Design review of the part built by this model. Coordinates are the model's own, in mm. Face numbers are marked on the shaded views. A direction names the side the tool comes from. Give positions to 0.01 mm unless a question says otherwise; leave off trailing zeros. Write each loop counter-clockwise with the first axis right and the second up, starting at its lowest first coordinate (ties: lowest second). Pieces come first, ordered by that corner, then holes. Notation, with made-up numbers: (89.25, 63.25) -> (99.25, 63.25) arc R22 ccw to (99.25, 97.25) -> close; hole circle Ø5 at (-33.5, 33.25). An arc over 180 degrees is marked (long way). Use CSV: the item, a comma, the result in double quotes.
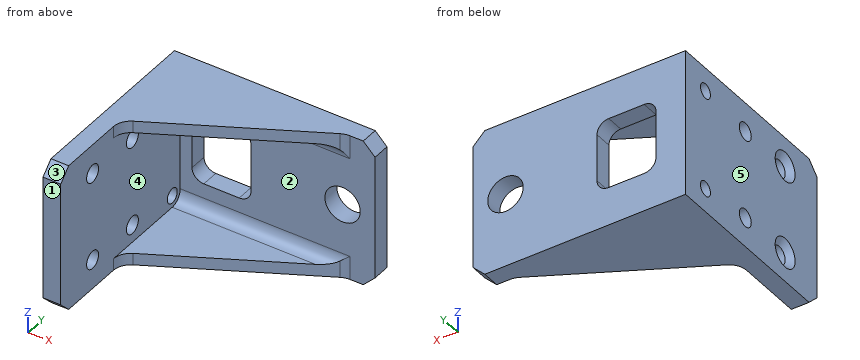
```python
from build123d import *

# Parameters (mm, degrees)
EXTRUDE_1_DEPTH     = 25
SKETCH_2_R          = 1.5
CUT_EXTRUDE_1_DEPTH = 55.863466897
HOLE_WIZARD_M3_1_D  = 2.5
CHAMFER_1_SIZE      = 1
SKETCH_5_R          = 3
CUT_EXTRUDE_2_DEPTH = 25
CUT_EXTRUDE_3_REACH = 56.863
SKETCH_6_W          = 10
SKETCH_6_H          = 12
FILLET_1_R          = 2
CHAMFER_2_SIZE      = 2
RIB_2_REACH         = 56.863
SKETCH_7_WALL_W     = 143.491694144
SKETCH_7_WALL_H     = 2
RIB_3_REACH         = 56.863
SKETCH_8_WALL_W     = 143.491694144
SKETCH_8_WALL_H     = 2
FILLET_2_R          = 2
FILLET_3_R          = 3


with BuildPart() as part:
    # 草图1 → 凸台-拉伸1 (new body)
    with BuildSketch(Plane.XY):
        Polygon((3, 30), (36, 30), (36, 33), (0, 33), (0, 0), (3, 0), align=None)
    extrude(amount=EXTRUDE_1_DEPTH)

    # 草图2 → 切除-拉伸1 (cut, through all)
    with BuildSketch(Plane.ZY):
        with Locations((5, 18)):
            Circle(SKETCH_2_R)
        with Locations((20, 18)):
            Circle(SKETCH_2_R)
        with Locations((20, 8)):
            Circle(SKETCH_2_R)
        with Locations((5, 8)):
            Circle(SKETCH_2_R)
    extrude(amount=-CUT_EXTRUDE_1_DEPTH, mode=Mode.SUBTRACT)

    # M3 螺纹孔1 (through all)
    with Locations(Plane(origin=(0, 28, 4), x_dir=(0, 0, -1), z_dir=(-1, 0, 0))):
        with Locations((0, 0), (-17, 0)):
            Hole(HOLE_WIZARD_M3_1_D / 2)

    # 倒角1
    chamfer_1_edges = [part.edges().sort_by_distance(p)[0] for p in [
        (0, 8, 18.5),
        (0, 8, 3.5),
    ]]
    chamfer(chamfer_1_edges, length=CHAMFER_1_SIZE)

    # 草图5 → 切除-拉伸2 (cut)
    with BuildSketch(Plane(origin=(0, 33, 0), x_dir=(1, 0, 0), z_dir=(0, 1, 0))):
        with Locations(Location((30.5, -12.5, 0), (0, 0, 180))):
            Circle(SKETCH_5_R)
    extrude(amount=-CUT_EXTRUDE_2_DEPTH, mode=Mode.SUBTRACT)

    # 草图6 → 切除-拉伸3 (cut, up to next)
    with BuildSketch(Plane(origin=(0, 33, 0), x_dir=(1, 0, 0), z_dir=(0, 1, 0)), mode=Mode.PRIVATE) as cut_extrude_3_sk1:
        with Locations((10, -12.5)):
            Rectangle(SKETCH_6_W, SKETCH_6_H)
    cut_extrude_3_tool1 = extrude(cut_extrude_3_sk1.sketch, amount=-CUT_EXTRUDE_3_REACH, mode=Mode.PRIVATE) & part.part
    add(cut_extrude_3_tool1.solids().sort_by_distance((10, 33, 12.5))[0], mode=Mode.SUBTRACT)

    # 圆角1
    fillet_1_edges = [part.edges().sort_by_distance(p)[0] for p in [
        (15, 31.5, 6.5),
        (15, 31.5, 18.5),
        (5, 31.5, 18.5),
        (5, 31.5, 6.5),
    ]]
    fillet(fillet_1_edges, radius=FILLET_1_R)

    # 倒角2
    chamfer_2_edges = [part.edges().sort_by_distance(p)[0] for p in [
        (36, 31.5, 25),
        (36, 31.5, 0),
        (1.5, 0, 25),
        (1.5, 0, 0),
    ]]
    chamfer(chamfer_2_edges, length=CHAMFER_2_SIZE)

    # 草图7 wall → 筋2 (add, up to next)
    with BuildSketch(Plane(origin=(17, 22.5, 25), x_dir=(0.881479970029, 0.472221412515, 0), z_dir=(-0.472221412515, 0.881479970029, 0)), mode=Mode.PRIVATE) as rib_2_sk1:
        with Locations((0, 1)):
            Rectangle(SKETCH_7_WALL_W, SKETCH_7_WALL_H)
    rib_2_tool1 = extrude(rib_2_sk1.sketch, amount=RIB_2_REACH, mode=Mode.PRIVATE) - part.part
    add(rib_2_tool1.solids().sort_by_distance((17, 22.5, 25))[0])

    # 草图8 wall → 筋3 (add, up to next)
    with BuildSketch(Plane(origin=(17, 22.5, 0), x_dir=(0.881479970029, 0.472221412515, 0), z_dir=(0.472221412515, -0.881479970029, 0)), mode=Mode.PRIVATE) as rib_3_sk1:
        with Locations((0, 1)):
            Rectangle(SKETCH_8_WALL_W, SKETCH_8_WALL_H)
    rib_3_tool1 = extrude(rib_3_sk1.sketch, amount=-RIB_3_REACH, mode=Mode.PRIVATE) - part.part
    add(rib_3_tool1.solids().sort_by_distance((17, 22.5, 0))[0])

    # 圆角2
    fillet_2_edges = [part.edges().sort_by_distance(p)[0] for p in [
        (17, 30, 23),
        (17, 30, 2),
    ]]
    fillet(fillet_2_edges, radius=FILLET_2_R)

    # 圆角3
    fillet_3_edges = [part.edges().sort_by_distance(p)[0] for p in [
        (31, 30, 2),
        (31, 30, 23),
        (3, 15, 24),
        (3, 15, 1),
    ]]
    fillet(fillet_3_edges, radius=FILLET_3_R)


solid = part.part
```
(1) Mouldability with a two-part tool opening along Z and no side actions: class the marked faces 1, 2 and 3 as +Z half, -Z half, draft (parallel to the pull), parting line (faces both ways), or undercut.
Established:
face 1,"draft"
face 2,"undercut"
face 3,"+Z half"
(2) Take a section at A-A (y = 18). Write out the cut boundary in (x, z).
Established:
outline,"(0, 0) -> (8.6, 0) -> (8.6, 2) -> (3, 2) -> (3, 3.5) -> (0, 3.5) -> close; (0, 6.5) -> (3, 6.5) -> (3, 18.5) -> (0, 18.5) -> close; (0, 21.5) -> (3, 21.5) -> (3, 23) -> (8.6, 23) -> (8.6, 25) -> (0, 25) -> close"
(3) Take a section at C-C (x = 24). Write out the cut boundary in (y, z), then the cut area to 3 significant figures.
Established:
outline,"(26.25, 0) -> (33, 0) -> (33, 25) -> (26.25, 25) -> (26.25, 23) -> (28, 23) arc R2 cw to (30, 21) -> (30, 4) arc R2 cw to (28, 2) -> (26.25, 2) -> close"
area,"91.7 mm2"
(4) Take a section at D-D (y = 25.5). Write out the cut boundary in (x, z).
Established:
outline,"(0, 0) -> (22.6, 0) -> (22.6, 2) -> (3, 2) -> (3, 23) -> (22.6, 23) -> (22.6, 25) -> (0, 25) -> close"
(5) Clearance check with flat-ended pins moving along their axes: pin 1 (4 mm diameter, centred on y = 25.5, z = 12, fed in from +X); pin 2 (8 mm diameter, centred on x = 23, z = 18, fed in from -Y); pin 3 (12.5 mm diameter, centred on x = 24.5, z = 12, fed in from -Y). State where each tip first meets the part, or that it passes through.
Established:
pin 1,"stops at x = 3"
pin 2,"stops at y = 29.73"
pin 3,"stops at y = 30"
(6) For line 1 along Z through (x, y) = (2.35, 28); line 2 along Z through (x, y) = (8, 18); line 3 along Y through (x, z) = (1.9, 5), list the stretches that pass through material, from the lowest coordinate up. Write a range as [from, to].
Established:
line 1,"z = [0, 2.75], [5.25, 19.75], [22.25, 25]"
line 2,"z = [0, 2], [23, 25]"
line 3,"y = [0, 6.5], [9.5, 16.5], [19.5, 27.25], [28.75, 33]"
(7) Tool access review of the marked faces 4 and 5: name each direction out of +Z, -Z, +X, -X, +Y, -Y from which nothing blocks a thin tool from reaching the whole face with its end or side.
Established:
face 4,"+X, -Y"
face 5,"+Z, -Z, -X, +Y, -Y"
(8) Take a section at B-B (z = 12.5). Write out the cut boundary in (x, y), then the cut area to 3 significant figures.
Established:
outline,"(0, 0) -> (3, 0) -> (3, 30) -> (5, 30) -> (5, 33) -> (0, 33) -> close; (15, 30) -> (27.5, 30) -> (27.5, 33) -> (15, 33) -> close; (33.5, 30) -> (36, 30) -> (36, 33) -> (33.5, 33) -> close"
area,"150 mm2"
